Geometry check sheet. Reference: the model listing, model coordinates, mm. A direction names the side the tool comes from. Coordinates: 2 decimals unless noted, no trailing zeros. Order: outer loops, then holes, each group sorted by start corner. A loop starts at its lowest first (then second) coordinate and runs counter-clockwise, first axis right, second up. Notation, with made-up numbers: (84, 7.25) - (109, 7.25) arc R29 ccw to (109, 29.25) - close; hole circle Ø1 at (22.5, -36.5). An arc over 180 degrees is marked (long way). Return JSON: item names as keys, results as strings. Group by question number.
Item 1: Section check C-C on z = -2.5. Enter the section's corners in (x, y), then the cut area to 3 significant figures.
Item 2: Draft check along Z on faces 1 (the flat face through (-18, -7, 1)), 2 (the flat face through (-18, 8, -1.75)), 3 (the cylindrical face through (1, 7.57, -0.05)). Enter one of: pulls with the +Z half, pulls with the -Z half, needs draft (parallel to the pull), parting line crosses it, or undercut.
Item 3: Section check B-B on y = 0. Enter the section's corners in (x, z), then the cut area to 3 significant figures.
Item 4: Gauge pin test, flat ends, axial feed: pin 1 (0.8 mm diameter, centred on x = -18, y = 8, fed in from -Z); pin 2 (2 mm diameter, centred on x = -17.5, y = -7, fed in from +Z); pin 3 (3 mm diameter, centred on x = -0.5, y = 5.5, fed in from -Z). Record the tip position at first contact, or that the pin passes through.
Item 5: Scan lines: probe 1 along Y at (x, z) = (-8.5, -0.25); probe 2 along X at (y, z) = (-0.75, -3); probe 3 along Y at (x, z) = (-2.25, -0.75). Record each from-to range of solid material in increasing order.
Item 6: Tool access check on faces 4 (the flat face through (-18, -8, -1.75)), 5 (the flat face through (-18, -7, 1.75)), 6 (the flat face through (-11, 6, -2)), 7 (the flat face through (-18, -7, -1)), 8 (the flat face through (-9, -9, 0)). Record the directions out of +Z, -Z, +X, -X, +Y, -Y that give a thin tool (end or side, any length) a straight path to the whole face; none if there is none.
Item 7: Section check D-D on z = 0. Enter the section's corners in (x, y), then the cut area to 3 significant figures.
Item 8: Section check A-A on x = -13.5. Enter the section's corners in (y, z).
from build123d import *

# Parameters (mm, degrees)
BOSS_EXTRUDE1_DEPTH     = 3.5
SKETCH2_R               = 0.6
CUT_EXTRUDE1_DEPTH      = 18.839562775
CUT_EXTRUDE2_DEPTH      = 26.347583711
BOSS_EXTRUDE3_START     = -18
SKETCH8_R               = 3
BOSS_EXTRUDE3_DEPTH     = 18
CUT_EXTRUDE6_DEPTH      = 23.321514286
CUT_EXTRUDE6_DEPTH_BACK = 23.321514286
SKETCH9_W               = 14.986497077
SKETCH9_H               = 12
CUT_EXTRUDE8_DEPTH      = 27.47640459
FILLET1_R               = 5


with BuildPart() as part:
    # Sketch1 → Boss-Extrude1 (new, symmetric)
    with BuildSketch(Plane.XY):
        with BuildLine():
            Line((-7.5, 6), (-17.5, 6))
            Line((-17.5, 6), (-17.5, 9))
            Line((-17.5, 9), (2.5, 9))
            Line((2.5, 9), (2.5, -9))
            Line((2.5, -9), (-4.576098932, -9))
            Line((-4.576098932, -9), (-17.5, -9))
            Line((-17.5, -9), (-17.5, -6))
            Line((-17.5, -6), (-7.5, -6))
            ThreePointArc((-7.5, -6), (-3.964466094, -4.535533906), (-2.5, -1))
            Line((-2.5, -1), (-2.5, 1))
            ThreePointArc((-2.5, 1), (-3.964466094, 4.535533906), (-7.5, 6))
        make_face()
    extrude(amount=BOSS_EXTRUDE1_DEPTH, both=True)

    # Sketch2 → Cut-Extrude1 (cut, through all)
    with BuildSketch(Plane.ZY.offset(2.5)):
        with Locations((1.5, 0)):
            Circle(SKETCH2_R)
        with Locations((-1.5, 0)):
            Circle(SKETCH2_R)
    extrude(amount=-CUT_EXTRUDE1_DEPTH, mode=Mode.SUBTRACT)

    # Sketch3 → Cut-Extrude2 (cut, through all)
    with BuildSketch(Plane(origin=(0, 9, 0), x_dir=(1, 0, 0), z_dir=(0, 1, 0))):
        with BuildLine():
            Line((-18.680784021, 1), (-16.328427125, 1))
            ThreePointArc((-16.328427125, 1), (-10.5, 0), (-16.328427125, -1))
            Line((-16.328427125, -1), (-18.680784021, -1))
            Line((-18.680784021, -1), (-18.680784021, 1))
        make_face()
    extrude(amount=-CUT_EXTRUDE2_DEPTH, mode=Mode.SUBTRACT)

    # Sketch8 → Boss-Extrude3 (add)
    with BuildSketch(Plane(origin=(0, 9, 0), x_dir=(1, 0, 0), z_dir=(0, 1, 0)).offset(BOSS_EXTRUDE3_START)):
        with BuildLine():
            Line((-17.372983346, 1), (-19, 1))
            Line((-19, 1), (-19, 1.75))
            Line((-19, 1.75), (-17.096873642, 1.75))
            ThreePointArc((-17.096873642, 1.75), (-9.5, 0), (-17.096873642, -1.75))
            Line((-17.096873642, -1.75), (-19, -1.75))
            Line((-19, -1.75), (-19, -1))
            Line((-19, -1), (-17.372983346, -1))
            ThreePointArc((-17.372983346, -1), (-17.5, 0), (-17.372983346, 1))
        make_face()
        with Locations(Location((-13.5, 0, 0), (0, 0, 180))):
            Circle(SKETCH8_R, mode=Mode.SUBTRACT)
    extrude(amount=BOSS_EXTRUDE3_DEPTH)

    # Sketch9 → Cut-Extrude6 (cut, two sides: drawn at the far end of the back side and taken through both)
    with BuildSketch(Plane(origin=(0, 0, -3.5), x_dir=(-1, 0, 0), z_dir=(0, 0, -1)).offset(-CUT_EXTRUDE6_DEPTH_BACK)):
        with Locations((14.993248539, 0)):
            Rectangle(SKETCH9_W, SKETCH9_H)
    extrude(amount=CUT_EXTRUDE6_DEPTH + CUT_EXTRUDE6_DEPTH_BACK, mode=Mode.SUBTRACT)

    # Sketch10 → Cut-Extrude8 (cut, through all)
    with BuildSketch(Plane(origin=(0, 9, 0), x_dir=(1, 0, 0), z_dir=(0, 1, 0))):
        with BuildLine():
            Line((-17.5, 1.75), (-17.096873642, 1.75))
            ThreePointArc((-17.096873642, 1.75), (-16.401750839, 2.753151298), (-15.436491673, 3.5))
            Line((-15.436491673, 3.5), (-17.5, 3.5))
            Line((-17.5, 3.5), (-17.5, 1.75))
        make_face()
        with BuildLine():
            Line((-17.5, -1.75), (-17.096873642, -1.75))
            ThreePointArc((-17.096873642, -1.75), (-16.401750839, -2.753151298), (-15.436491673, -3.5))
            Line((-15.436491673, -3.5), (-17.5, -3.5))
            Line((-17.5, -3.5), (-17.5, -1.75))
        make_face()
        with BuildLine():
            Line((-17.372983346, -1), (-16.328427125, -1))
            ThreePointArc((-16.328427125, -1), (-16.5, 0), (-16.328427125, 1))
            Line((-16.328427125, 1), (-17.372983346, 1))
            ThreePointArc((-17.372983346, 1), (-17.5, 0), (-17.372983346, -1))
        make_face()
    extrude(amount=-CUT_EXTRUDE8_DEPTH, mode=Mode.SUBTRACT)

    # Fillet1
    fillet1_edges = [part.edges().sort_by_distance(p)[0] for p in [
        (2.5, 9, 0),
        (2.5, -9, 0),
    ]]
    fillet(fillet1_edges, radius=FILLET1_R)


solid = part.part
Computed:
{
 "1": {"outline": "(-16.62, -9) - (-15.16, -9) - (-15.16, -6) - (-16.62, -6) - close; (-16.62, 6) - (-15.16, 6) - (-15.16, 9) - (-16.62, 9) - close; (-11.84, -9) - (-2.5, -9) arc R5 ccw to (2.5, -4) - (2.5, 4) arc R5 ccw to (-2.5, 9) - (-11.84, 9) - (-11.84, 6) - (-7.5, 6) arc R5 cw to (-2.5, 1) - (-2.5, -1) arc R5 cw to (-7.5, -6) - (-11.84, -6) - close", "area": "155 mm²"},
 "2": {"face 1": "undercut", "face 2": "pulls with the -Z half", "face 3": "needs draft"},
 "3": {"outline": "(-2.5, -3.5) - (2.5, -3.5) - (2.5, -2.1) - (-2.5, -2.1) - close; (-2.5, -0.9) - (2.5, -0.9) - (2.5, 0.9) - (-2.5, 0.9) - close; (-2.5, 2.1) - (2.5, 2.1) - (2.5, 3.5) - (-2.5, 3.5) - close", "area": "23.0 mm²"},
 "4": {"pin 1": "stops at z = -1.75", "pin 2": "stops at z = 2.65", "pin 3": "stops at z = -3.5"},
 "5": {"probe 1": "y = -9 to -6, 6 to 9", "probe 2": "x = -2.5 to 2.5", "probe 3": "y = -8.99 to 8.99"},
 "6": {"face 4": "-Z, -X, +Y, -Y", "face 5": "+Z, -X, +Y, -Y", "face 6": "+Z, -Z, -X", "face 7": "-X, +Y, -Y", "face 8": "+Z, -Z, +X, -X, -Y"},
 "7": {"outline": "(-10.5, -9) - (-2.5, -9) arc R5 ccw to (2.5, -4) - (2.5, 4) arc R5 ccw to (-2.5, 9) - (-10.5, 9) - (-10.5, 6) - (-7.5, 6) arc R5 cw to (-2.5, 1) - (-2.5, -1) arc R5 cw to (-7.5, -6) - (-10.5, -6) - close", "area": "138 mm²"},
 "8": {"outline": "(-9, -4) - (-6, -4) - (-6, -3) - (-9, -3) - close; (-9, 3) - (-6, 3) - (-6, 4) - (-9, 4) - close; (6, -4) - (9, -4) - (9, -3) - (6, -3) - close; (6, 3) - (9, 3) - (9, 4) - (6, 4) - close"}
}
